Geometry: final body of the model. Coordinates: model frame, mm. A direction names the side the tool comes from. Coordinates: 2 decimals unless noted, no trailing zeros. Loops run counter-clockwise (first coordinate to the right, second up) from the corner with the lowest first, then second, coordinate; pieces in that order, holes last. Notation, with made-up numbers: (31, 55.5) - (64, 55.5) arc R26 cw to (64, 81.5) - close; hole circle Ø3 at (39, -32.5). An arc over 180 degrees is marked (long way). Write each question's results on one line, items separated by ' | '. Start each with the question number.
from build123d import *

# Parameters (mm, degrees)
ESBO_O1_R                = 1.6
RESSALTO_EXTRUS_O1_DEPTH = 3
FILETE1_R                = 10
FILETE2_START            = -1
FILETE2_DEPTH            = 5
FILETE2_2_DEPTH          = 3


with BuildPart() as part:
    # Esboço1 → Ressalto-extrusão1 (new body)
    with BuildSketch(Plane.XY):
        Polygon((-31.75, -26.93380815), (-18.341364608, -45.93380815), (18.341364608, -45.93380815), (31.75, -26.93380815), (31.75, 17.5), (-31.75, 17.5), align=None)
        with Locations((-12.806248475, -36.43380815)):
            Circle(ESBO_O1_R, mode=Mode.SUBTRACT)
        with Locations((12.806248475, -36.43380815)):
            Circle(ESBO_O1_R, mode=Mode.SUBTRACT)
        with Locations((-24.75, -5)):
            Circle(ESBO_O1_R, mode=Mode.SUBTRACT)
        with Locations((-24.75, 5)):
            Circle(ESBO_O1_R, mode=Mode.SUBTRACT)
        with BuildLine():
            Line((-18, 12.5), (18, 12.5))
            ThreePointArc((18, 12.5), (19.767766953, 11.767766953), (20.5, 10))
            Line((20.5, 10), (20.5, 2.5))
            Line((20.5, 2.5), (26.75, 2.5))
            Line((26.75, 2.5), (26.75, -2.5))
            Line((26.75, -2.5), (20.5, -2.5))
            Line((20.5, -2.5), (20.5, -10))
            ThreePointArc((20.5, -10), (19.767766953, -11.767766953), (18, -12.5))
            Line((18, -12.5), (-18, -12.5))
            ThreePointArc((-18, -12.5), (-19.767766953, -11.767766953), (-20.5, -10))
            Line((-20.5, -10), (-20.5, -2.5))
            Line((-20.5, -2.5), (-26.75, -2.5))
            Line((-26.75, -2.5), (-26.75, 2.5))
            Line((-26.75, 2.5), (-20.5, 2.5))
            Line((-20.5, 2.5), (-20.5, 10))
            ThreePointArc((-20.5, 10), (-19.767766953, 11.767766953), (-18, 12.5))
        make_face(mode=Mode.SUBTRACT)
        with Locations((24.75, -5)):
            Circle(ESBO_O1_R, mode=Mode.SUBTRACT)
        with Locations((24.75, 5)):
            Circle(ESBO_O1_R, mode=Mode.SUBTRACT)
    extrude(amount=RESSALTO_EXTRUS_O1_DEPTH)

    # Filete1
    filete1_edges = [part.edges().sort_by_distance(p)[0] for p in [
        (-31.75, 17.5, 1.5),
        (31.75, 17.5, 1.5),
        (31.75, -26.93380815, 1.5),
        (18.341364608, -45.93380815, 1.5),
        (-18.341364608, -45.93380815, 1.5),
        (-31.75, -26.93380815, 1.5),
    ]]
    fillet(filete1_edges, radius=FILETE1_R)

    # Filete2: read off the stored shape, not the designer's step
    # Filete2 outline → Filete2 (cut)
    with BuildSketch(Plane.XY.offset(FILETE2_START)):
        with BuildLine():
            Line((-20.5, -2.5), (-23, -2.5))
            ThreePointArc((-23, -2.5), (-21.232233047, -3.232233047), (-20.5, -5))
            Line((-20.5, -5), (-20.5, -2.5))
        make_face()
        with BuildLine():
            ThreePointArc((-20.5, 5), (-21.232233047, 3.232233047), (-23, 2.5))
            Line((-23, 2.5), (-20.5, 2.5))
            Line((-20.5, 2.5), (-20.5, 5))
        make_face()
        with BuildLine():
            Line((20.5, -2.5), (20.5, -5))
            ThreePointArc((20.5, -5), (21.232233047, -3.232233047), (23, -2.5))
            Line((23, -2.5), (20.5, -2.5))
        make_face()
        with BuildLine():
            Line((20.5, 2.5), (23, 2.5))
            ThreePointArc((23, 2.5), (21.232233047, 3.232233047), (20.5, 5))
            Line((20.5, 5), (20.5, 2.5))
        make_face()
    extrude(amount=FILETE2_DEPTH, mode=Mode.SUBTRACT)

    # Filete2 2 outline → Filete2 2 (add)
    with BuildSketch(Plane.XY):
        with BuildLine():
            ThreePointArc((-24.25, -2.5), (-26.017766953, -1.767766953), (-26.75, 0))
            Line((-26.75, 0), (-26.75, -2.5))
            Line((-26.75, -2.5), (-24.25, -2.5))
        make_face()
        with BuildLine():
            ThreePointArc((-26.75, 0), (-26.017766953, 1.767766953), (-24.25, 2.5))
            Line((-24.25, 2.5), (-26.75, 2.5))
            Line((-26.75, 2.5), (-26.75, 0))
        make_face()
        with BuildLine():
            ThreePointArc((24.25, 2.5), (26.017766953, 1.767766953), (26.75, 0))
            Line((26.75, 0), (26.75, 2.5))
            Line((26.75, 2.5), (24.25, 2.5))
        make_face()
        with BuildLine():
            ThreePointArc((26.75, 0), (26.017766953, -1.767766953), (24.25, -2.5))
            Line((24.25, -2.5), (26.75, -2.5))
            Line((26.75, -2.5), (26.75, 0))
        make_face()
    extrude(amount=FILETE2_2_DEPTH)


solid = part.part
1) Pull-direction query (Y, two-part tool) for faces 1 (the flat face through (25.565, -35.698, 1.479)), 2 (the cylindrical face through (25.49, 3.58, 1.48)), 3 (the cylindrical face through (28.74, 14.65, 1.52)); classes: released by +Y, released by -Y, zero draft, split by the parting line, or undercut.
2) Pin query (flat end, axial travel): pin 1 Ø3.5 at (x, y) = (12.81, -36.43) entering from -Z; pin 2 Ø2.5 at (x, y) = (24.75, 5) entering from +Z; pin 3 Ø1 at (x, z) = (23.5, 1.5) entering from -Y; pin 4 Ø1 at (x, z) = (-24, 1.5) entering from +Y. Return the tip coordinate at first contact, or that it passes through.
3) Section query B-B on y = 11. Output: boundary loops of the cut face in (x, z).
4) Material intervals for line 1 (Y direction, x = 13, z = 2.5); line 2 (Y direction, x = -10.5, z = 1.1); line 3 (Y direction, x = 24.75, z = 1.6), sorted ascending. Write a range as [from, to].
5) Section query A-A on x = 4.5. Output: boundary loops of the cut face in (y, z).
6) Access query for faces 4 (the cylindrical face through (-21.213, 3.252, 1.479)), 5 (the cylindrical face through (17.701, -44.843, 1.521)). Directions: +Z, -Z, +X, -X, +Y, -Y. A direction counts if a zero-diameter tool reaches every point of the face in a straight line with its end or side. Return the directions, or none.
7) Section query C-C on z = 2.3. Count the separate pieces of the cut face and the enclosed holes in it, and give its area (3 significant figures).
Returned:
1) face 1: released by -Y | face 2: undercut | face 3: released by +Y
2) pin 1: stops at z = 0 | pin 2: passes through | pin 3: stops at y = -39.33 | pin 4: stops at y = 17.35
3) outline: (-31.12, 0) - (-20.29, 0) - (-20.29, 3) - (-31.12, 3) - close; (20.29, 0) - (31.12, 0) - (31.12, 3) - (20.29, 3) - close
4) line 1: y = [-45.93, -38.02], [-34.85, -12.5], [12.5, 17.5] | line 2: y = [-45.93, -12.5], [12.5, 17.5] | line 3: y = [-36.85, -6.6], [-3.4, -2.45], [2.45, 3.4], [6.6, 17.04]
5) outline: (-45.93, 0) - (-12.5, 0) - (-12.5, 3) - (-45.93, 3) - close; (12.5, 0) - (17.5, 0) - (17.5, 3) - (12.5, 3) - close
6) face 4: +Z, -Z | face 5: +Z, -Z, +X, -Y
7) separate pieces: 1 | enclosed holes: 7 | area: 2,590 mm²
